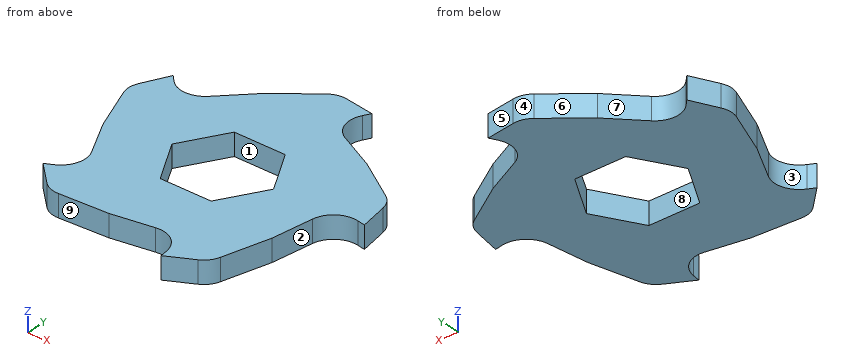
```python
from build123d import *

# Parameters (mm, degrees)
SKETCH1_R           = 125
BOSS_EXTRUDE1_DEPTH = 20
CUT_EXTRUDE1_START  = -30
CUT_EXTRUDE1_DEPTH  = 30


with BuildPart() as part:
    # Sketch1 → Boss-Extrude1 (new body)
    with BuildSketch(Plane.XY):
        Circle(SKETCH1_R)
        Polygon((23.094010768, -40), (46.188021535, 0), (23.094010768, 40), (-23.094010768, 40), (-46.188021535, 0), (-23.094010768, -40), align=None, mode=Mode.SUBTRACT)
    extrude(amount=BOSS_EXTRUDE1_DEPTH)

    # Sketch3 → Cut-Extrude1 (cut)
    with BuildSketch(Plane.XY.offset(20).offset(CUT_EXTRUDE1_START)):
        with BuildLine():
            ThreePointArc((-6.774110793, 119.467271802), (0.492536101, 123.239201876), (8.661716474, 123.783357737))
            Line((8.661716474, 123.783357737), (34.45, 120.159050845))
            ThreePointArc((34.45, 120.159050845), (-42.75708256, 117.459916103), (-103.632412842, 69.895085725))
            Line((-103.632412842, 69.895085725), (-98.652289989, 64.738017545))
            ThreePointArc((-98.652289989, 64.738017545), (-82.862560201, 58.020530735), (-67.051084533, 64.686671523))
            Line((-67.051084533, 64.686671523), (-40.898801445, 91.592627068))
            Line((-40.898801445, 91.592627068), (-6.774110793, 119.467271802))
        make_face()
        with BuildLine():
            ThreePointArc((124.923683754, 4.367291753), (98.498353472, 76.96151222), (34.45, 120.159050845))
            Line((34.45, 120.159050845), (31.084279298, 113.829050845))
            ThreePointArc((31.084279298, 113.829050845), (29.574864535, 96.736307856), (40.800755858, 83.75865168))
            Line((40.800755858, 83.75865168), (74.471340122, 67.200749946))
            Line((74.471340122, 67.200749946), (111.526811975, 43.35997947))
            ThreePointArc((111.526811975, 43.35997947), (117.359648033, 37.614578084), (120.401586576, 30.013379267))
            Line((120.401586576, 30.013379267), (124.923683754, 4.367291753))
        make_face()
        with BuildLine():
            ThreePointArc((42.75708256, -117.459916103), (103.632412842, -69.895085725), (124.923683754, 4.367291753))
            Line((124.923683754, 4.367291753), (117.863431111, 5.612204784))
            ThreePointArc((117.863431111, 5.612204784), (101.140831696, 1.765795466), (92.26733842, -12.920977933))
            Line((92.26733842, -12.920977933), (86.924620828, -50.060279532))
            Line((86.924620828, -50.060279532), (75.70147125, -92.669330738))
            ThreePointArc((75.70147125, -92.669330738), (72.039715291, -99.992114147), (65.75055633, -105.234069233))
            Line((65.75055633, -105.234069233), (42.75708256, -117.459916103))
        make_face()
        with BuildLine():
            Line((-115.048351394, 46.488943056), (-103.632412842, 69.895085725))
            ThreePointArc((-103.632412842, 69.895085725), (-124.923683754, -4.367291753), (-98.498353472, -76.96151222))
            Line((-98.498353472, -76.96151222), (-92.054747579, -73.818755638))
            ThreePointArc((-92.054747579, -73.818755638), (-80.786743134, -60.877647816), (-82.240605082, -43.780090059))
            Line((-82.240605082, -43.780090059), (-99.748189513, -10.593393299))
            Line((-99.748189513, -10.593393299), (-115.713442688, 30.474855047))
            ThreePointArc((-115.713442688, 30.474855047), (-117.055243981, 38.551437421), (-115.048351394, 46.488943056))
        make_face()
        with BuildLine():
            Line((-79.765507985, -95.051610828), (-98.498353472, -76.96151222))
            ThreePointArc((-98.498353472, -76.96151222), (-34.45, -120.159050845), (42.75708256, -117.459916103))
            Line((42.75708256, -117.459916103), (41.75932716, -110.360517537))
            ThreePointArc((41.75932716, -110.360517537), (32.933607104, -95.644986241), (16.223595337, -91.744255211))
            Line((16.223595337, -91.744255211), (-20.748969991, -98.139704183))
            Line((-20.748969991, -98.139704183), (-64.740729744, -100.632775581))
            ThreePointArc((-64.740729744, -100.632775581), (-72.836655443, -99.413103234), (-79.765507985, -95.051610828))
        make_face()
    extrude(amount=CUT_EXTRUDE1_DEPTH, mode=Mode.SUBTRACT)


solid = part.part
```
Build history of the part. All positions in model axes, mm. Face numbers are marked on the shaded views. A direction names the side the tool comes from. Coordinates: 2 decimals unless noted, no trailing zeros. Order: outer loops, then holes, each group sorted by start corner. A loop starts at its lowest first (then second) coordinate and runs counter-clockwise, first axis right, second up. Notation, with made-up numbers: M 86.25,20.25 L 97.25,20.25 A26 cw 97.25,38.25 Z; hole C 72,-37 d4. An arc over 180 degrees is marked long. One line per question, with ' | ' between items. Start each with the question number.
1. Cut at B-B (y = 37). Write the cut outline in (x, z).
2. Cut at D-D (x = 55). Write the cut outline in (y, z).
3. Flat gauge pins, fed straight in: P1, Ø3, axis at x = 91, z = 15, coming from the +Y side; P2, Ø1.5, axis at x = 88.5, z = 2.5, coming from the +Y side; P3, Ø1.5, axis at y = 72.5, z = 13.5, coming from the -X side. Where does each tip first touch, or does it go through?
4. Mould opens along Y. For the marked faces 1, 2, 3 and 4 say: +Y half, -Y half, draft (parallel to the pull), parting line (faces both ways), or undercut.
5. Cut at A-A (x = -10.5). Write the cut outline in (y, z).
6. Tool access for the marked faces 5, 6, 7, 8 and 9: list every direction of +Z, -Z, +X, -X, +Y, -Y with a clear straight run to the whole face (end or side of a thin tool).
7. Cut at C-C (y = 76). Write the cut outline in (x, z).
8. Wall check: line 1 along Y through (x, z) = (21, 3.5); line 2 along X through (y, z) = (-35, 18); line 3 along X through (y, z) = (-37, 17.5). Give the ranges that are in metal, low to high. Write a range as [from, to].
The answers:
1) outline: M -117.06,0 L -24.83,0 L -24.83,20 L -117.06,20 Z; M 24.83,0 L 117.75,0 L 117.75,20 L 24.83,20 Z
2) outline: M -110.95,0 L 76.78,0 L 76.78,20 L -110.95,20 Z
3) P1: stops at y = 57.53 | P2: stops at y = 58.66 | P3: stops at x = -60.19
4) face 1: undercut | face 2: -Y half | face 3: undercut | face 4: +Y half
5) outline: M -96.37,0 L -40,0 L -40,20 L -96.37,20 Z; M 40,0 L 116.42,0 L 116.42,20 L 40,20 Z
6) face 5: +Z, -Z, +X, +Y | face 6: +Z, -Z, -X, +Y | face 7: +Z, -Z, +Y | face 8: +Z, -Z | face 9: +Z, -Z, -Y
7) outline: M -56.05,0 L 56.58,0 L 56.58,20 L -56.05,20 Z
8) line 1: y = [-91.45, -40], [40, 122.05] | line 2: x = [-86.87, -25.98], [25.98, 89.09] | line 3: x = [-85.82, -24.83], [24.83, 88.8]
